Design review of the part built by this model. Coordinates are the model's own, in mm. Coordinates: 2 decimals unless noted, no trailing zeros. Write each loop counter-clockwise with the first axis right and the second up, starting at its lowest first coordinate (ties: lowest second). Pieces come first, ordered by that corner, then holes. Notation, with made-up numbers: (17, 66.25) - (48, 66.25) arc R11 cw to (48, 81.25) - close; hole circle Ø8 at (-19.5, 34). An arc over 180 degrees is marked (long way). Use a Markdown table: item, result.
from build123d import *

# Parameters (mm, degrees)
BOSS_EXTRUDE1_DEPTH = 24
FILLET1_R           = 1


with BuildPart() as part:
    # Sketch1 → Boss-Extrude1 (new body)
    with BuildSketch(Plane.XY):
        with BuildLine():
            ThreePointArc((94, 0), (93.625231148, 1.690473047), (92.571150439, 3.064177772))
            ThreePointArc((92.571150439, 3.064177772), (86, 0), (92.571150439, -3.064177772))
            ThreePointArc((92.571150439, -3.064177772), (93.625231148, -1.690473047), (94, 0))
        make_face()
    extrude(amount=BOSS_EXTRUDE1_DEPTH)

    # Fillet1
    fillet1_edges = [part.edges().sort_by_distance(p)[0] for p in [
        (87.428849561, 3.064177772, 0),
        (87.428849561, 3.064177772, 24),
    ]]
    fillet(fillet1_edges, radius=FILLET1_R)


solid = part.part
(1) Take a section at A-A on z = 18.25. Write out the cut boundary in (x, y).
Determined:
| item | result |
|---|---|
| outline | circle Ø8 at (90, 0) |
(2) For pin 1 (4 mm diameter, centred on x = 89.5, z = 3, fed in from -Y), flat-tipped, find the tip position at first contact; note if it passes through.
Determined:
| item | result |
|---|---|
| pin 1 | y = -4 |
(3) For L1, parallel to X at y = 1.25, z = 21; L2, parallel to Y at x = 86.5, z = 8.5; L3, parallel to Y at x = 91, z = 6.75, list the stretches that pass through material, from the lowest coordinate up. Write a range as from..to.
Determined:
| item | result |
|---|---|
| L1 | 86.2..93.8 |
| L2 | -1.94..1.94 |
| L3 | -3.87..3.87 |
